Read the model definition and answer for the solid it produces. Units are mm, in the model's axes. Face numbers are marked on the shaded views. A direction names the side the tool comes from. Round coordinates to 2 decimals unless told otherwise and drop trailing zeros. Order: outer loops, then holes, each group sorted by start corner. A loop starts at its lowest first (then second) coordinate and runs counter-clockwise, first axis right, second up. Notation, with made-up numbers: (28, -34.75) -> (42, -34.75) arc R32 ccw to (42, 4.25) -> close; hole circle Ø7 at (21.25, -17.5). An arc over 180 degrees is marked (long way). Answer as a JSON object with one key per item and string values. Group by question number.
Item 1: Given P1, Ø1.5, axis at x = 36.5, y = 53, coming from the +Z side; P2, Ø1.2, axis at x = 68, z = 1.5, coming from the +Y side; P3, Ø5.5, axis at x = 5, y = 61.58, coming from the -Z side; P4, Ø6, axis at x = 69.34, y = 19, coming from the +Z side, each flat-ended and moving along its own axis, determine where each tip first touches the part or whether it passes through.
Item 2: Section A-A, the plane x = 60 is taken. Write down the section's boundary in (y, z).
Item 3: Section B-B, the plane y = 53.45 is taken. Count the separate pieces of the cut face and the enclosed holes in it, plus the area to 3 significant figures.
Item 4: Consider probe 1 along Y at (x, z) = (37.17, 4.75); probe 2 along Z at (x, y) = (67, 32.5); probe 3 along Y at (x, z) = (69.34, 10.5). Determine where each line is inside the solid, lowest interval first. Write a range as from..to.
Item 5: The mould has two halves that part along X. Classify the marked faces 1, 2, 3 and 4: pulls with the +X half, pulls with the -X half, needs draft (parallel to the pull), parting line crosses it, or undercut.
Item 6: For the marked faces 5, 6 and 7, determine the directions among +Z, -Z, +X, -X, +Y, -Y from which every point of the face is accessible in a straight line to the end or side of a thin tool.
Item 7: Section D-D, the plane x = 37.17 is taken. Write down the section's boundary in (y, z).
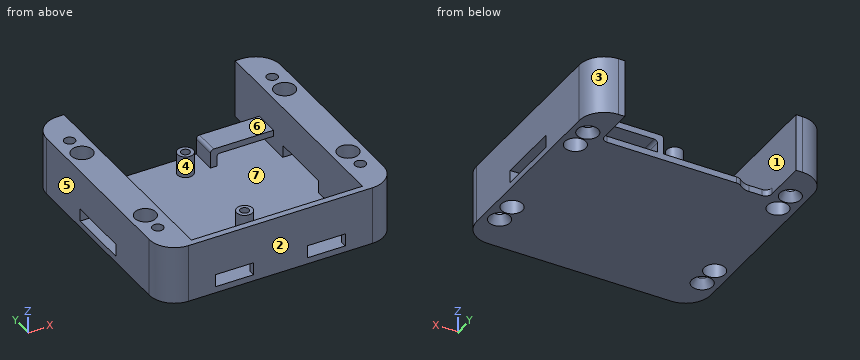
from build123d import *

# Parameters (mm, degrees)
F1_R      = 1.75
F1_R_2    = 3.35
F2_DEPTH  = 2
F3_R      = 2
F4_R      = 1.75
F4_R_2    = 3.35
F5_DEPTH  = 16.51
F6_SIZE2  = 2.8
F6_SIZE   = 1.6
F7_R      = 2.5
F7_R_2    = 1.4
F8_DEPTH  = 6.85
F9_W      = 20
F9_H      = 4
F10_DEPTH = 10.001
F11_W     = 20
F11_H     = 4
F12_DEPTH = 10.001
F13_W     = 12
F13_H     = 4
F14_DEPTH = 2.001
F15_W     = 20
F15_H     = 8
F16_DEPTH = 6
F17_W     = 18
F17_H     = 4
F18_DEPTH = 8
F19_R     = 1


with BuildPart() as f2:
    # F1 (on Top) → F2 (new body)
    with BuildSketch(Plane.XY):
        with BuildLine():
            ThreePointArc((8, 73.58), (2.343146, 71.236854), (0, 65.58))
            Line((0, 65.58), (0, 8))
            ThreePointArc((0, 8), (2.343146, 2.343146), (8, 0))
            Line((8, 0), (66.34, 0))
            ThreePointArc((66.34, 0), (71.996854, 2.343146), (74.34, 8))
            Line((74.34, 8), (74.34, 65.58))
            ThreePointArc((74.34, 65.58), (71.996854, 71.236854), (66.34, 73.58))
            Line((66.34, 73.58), (64.34, 73.58))
            Line((64.34, 73.58), (64.34, 59.98))
            Line((64.34, 59.98), (21.181552, 59.98))
            ThreePointArc((21.181552, 59.98), (20.280164, 59.811845), (19.500034, 59.33))
            ThreePointArc((19.500034, 59.33), (17.939776, 58.36631), (16.137, 58.03))
            Line((16.137, 58.03), (10, 58.03))
            Line((10, 58.03), (10, 73.58))
            Line((10, 73.58), (8, 73.58))
        make_face()
        with Locations((5, 12)):
            Circle(F1_R, mode=Mode.SUBTRACT)
        with Locations((5, 19)):
            Circle(F1_R_2, mode=Mode.SUBTRACT)
        with Locations((69.34, 12)):
            Circle(F1_R, mode=Mode.SUBTRACT)
        with Locations((69.34, 19)):
            Circle(F1_R_2, mode=Mode.SUBTRACT)
        with Locations((5, 54.58)):
            Circle(F1_R_2, mode=Mode.SUBTRACT)
        with Locations((5, 61.58)):
            Circle(F1_R, mode=Mode.SUBTRACT)
        with Locations((69.34, 54.58)):
            Circle(F1_R_2, mode=Mode.SUBTRACT)
        with Locations((69.34, 61.58)):
            Circle(F1_R, mode=Mode.SUBTRACT)
    extrude(amount=-F2_DEPTH)

    # F3
    f3_edges = [f2.edges().sort_by_distance(p)[0] for p in [
        (10, 58.03, -1),
        (64.34, 59.98, -1),
    ]]
    fillet(f3_edges, radius=F3_R)

    # F4 (on face) → F5 (join)
    with BuildSketch(Plane.XY):
        with BuildLine():
            ThreePointArc((8, 73.58), (2.343146, 71.236854), (0, 65.58))
            Line((0, 65.58), (0, 8))
            ThreePointArc((0, 8), (2.343146, 2.343146), (8, 0))
            Line((8, 0), (66.34, 0))
            ThreePointArc((66.34, 0), (71.996854, 2.343146), (74.34, 8))
            Line((74.34, 8), (74.34, 65.58))
            ThreePointArc((74.34, 65.58), (71.996854, 71.236854), (66.34, 73.58))
            Line((66.34, 73.58), (64.34, 73.58))
            Line((64.34, 73.58), (64.34, 2))
            Line((64.34, 2), (10, 2))
            Line((10, 2), (10, 73.58))
            Line((10, 73.58), (8, 73.58))
        make_face()
        with Locations((5, 12)):
            Circle(F4_R, mode=Mode.SUBTRACT)
        with Locations((5, 19)):
            Circle(F4_R_2, mode=Mode.SUBTRACT)
        with Locations((69.34, 12)):
            Circle(F4_R, mode=Mode.SUBTRACT)
        with Locations((69.34, 19)):
            Circle(F4_R_2, mode=Mode.SUBTRACT)
        with Locations((5, 54.58)):
            Circle(F4_R_2, mode=Mode.SUBTRACT)
        with Locations((5, 61.58)):
            Circle(F4_R, mode=Mode.SUBTRACT)
        with Locations((69.34, 54.58)):
            Circle(F4_R_2, mode=Mode.SUBTRACT)
        with Locations((69.34, 61.58)):
            Circle(F4_R, mode=Mode.SUBTRACT)
    extrude(amount=F5_DEPTH)

    # F6
    f6_edges = [f2.edges().sort_by_distance(p)[0] for p in [
        (3.25, 61.58, -2),
        (3.25, 12, -2),
        (67.59, 12, -2),
        (67.59, 61.58, -2),
    ]]
    chamfer(f6_edges, length=F6_SIZE, length2=F6_SIZE2)

    # F7 (on face) → F8 (join)
    with BuildSketch(Plane.XY):
        with Locations((37.17, 53.45)):
            Circle(F7_R)
        with Locations((37.17, 53.45)):
            Circle(F7_R_2, mode=Mode.SUBTRACT)
        with Locations((37.17, 20.13)):
            Circle(F7_R)
        with Locations((37.17, 20.13)):
            Circle(F7_R_2, mode=Mode.SUBTRACT)
    extrude(amount=F8_DEPTH)

    # F9 (on face) → F10 (cut, through all)
    with BuildSketch(Plane.YZ.offset(10)):
        with Locations((36.79, 2)):
            Rectangle(F9_W, F9_H)
    extrude(amount=-F10_DEPTH, mode=Mode.SUBTRACT)

    # F11 (on face) → F12 (cut, through all)
    with BuildSketch(Plane(origin=(64.34, 0, 0), x_dir=(0, -1, 0), z_dir=(-1, 0, 0))):
        with Locations((-36.79, 2)):
            Rectangle(F11_W, F11_H)
    extrude(amount=-F12_DEPTH, mode=Mode.SUBTRACT)

    # F13 (on face) → F14 (cut, through all)
    with BuildSketch(Plane(origin=(0, 2, 0), x_dir=(-1, 0, 0), z_dir=(0, 1, 0))):
        with Locations((-51.755, 2)):
            Rectangle(F13_W, F13_H)
        with Locations((-22.585, 2)):
            Rectangle(F13_W, F13_H)
    extrude(amount=-F14_DEPTH, mode=Mode.SUBTRACT)

    # F15 (on face) → F16 (join)
    with BuildSketch(Plane.XY):
        with Locations((54.34, 55.98)):
            Rectangle(F15_W, F15_H)
    extrude(amount=F16_DEPTH)

    # F17 (on face) → F18 (cut, through all)
    with BuildSketch(Plane(origin=(0, 59.98, 0), x_dir=(-1, 0, 0), z_dir=(0, 1, 0))):
        with Locations((-55.34, 2)):
            Rectangle(F17_W, F17_H)
    extrude(amount=-F18_DEPTH, mode=Mode.SUBTRACT)

    # F19
    f19_edges = [f2.edges().sort_by_distance(p)[0] for p in [
        (46.34, 55.98, 4),
        (44.34, 55.98, 6),
    ]]
    fillet(f19_edges, radius=F19_R)


solid = f2.part
Values found:
{
 "1": {"P1": "z = 6.85", "P2": "y = 73.51", "P3": "z = -0.95", "P4": "through"},
 "2": {"outline": "(0, -2) -> (59.98, -2) -> (59.98, 0) -> (2, 0) -> (2, 16.51) -> (0, 16.51) -> close; (51.98, 4) -> (59.98, 4) -> (59.98, 6) -> (51.98, 6) -> close"},
 "3": {"separate pieces": "3", "enclosed holes": "1", "area": "308 mm2"},
 "4": {"probe 1": "0..2, 17.63..18.73, 21.53..22.63, 50.95..52.05, 54.85..55.95", "probe 2": "-2..0, 4..16.51", "probe 3": "0.58..10.25, 13.75..15.65, 22.35..51.23, 57.93..59.83, 63.33..73"},
 "5": {"face 1": "undercut", "face 2": "needs draft", "face 3": "pulls with the +X half", "face 4": "undercut"},
 "6": {"face 5": "+Z, -Z, -X, +Y, -Y", "face 6": "+Z, +Y", "face 7": "none"},
 "7": {"outline": "(0, -2) -> (59.98, -2) -> (59.98, 0) -> (55.95, 0) -> (55.95, 6.85) -> (54.85, 6.85) -> (54.85, 0) -> (52.05, 0) -> (52.05, 6.85) -> (50.95, 6.85) -> (50.95, 0) -> (22.63, 0) -> (22.63, 6.85) -> (21.53, 6.85) -> (21.53, 0) -> (18.73, 0) -> (18.73, 6.85) -> (17.63, 6.85) -> (17.63, 0) -> (2, 0) -> (2, 16.51) -> (0, 16.51) -> close"}
}
